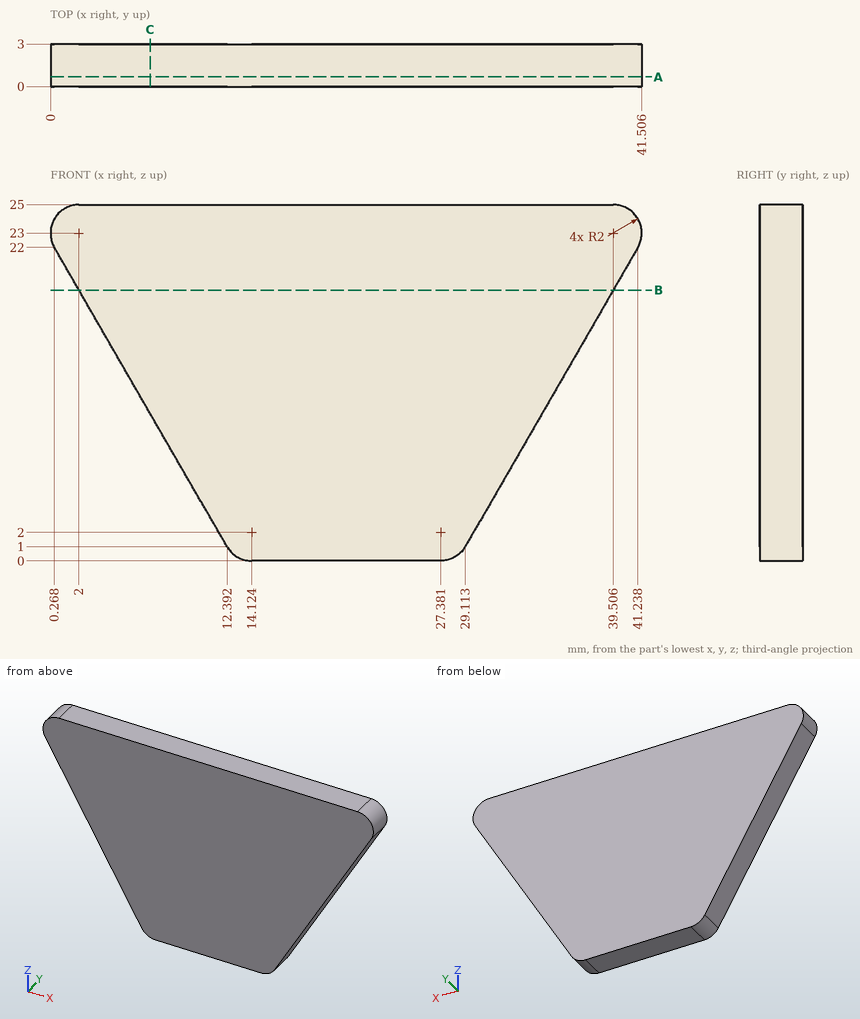
Design review of the part shown in the three views and the two pictorial views. Dimensions are in mm from the part's minimum x, y and z. Round coordinates to 2 decimals unless told otherwise and drop trailing zeros. Loops run counter-clockwise (first coordinate to the right, second up) from the corner with the lowest first, then second, coordinate; pieces in that order, holes last. Notation, with made-up numbers: (48.5, -2.75) - (105.5, -2.75) arc R16 ccw to (105.5, 5.25) - close; hole circle Ø9 at (22, -35). An arc over 180 degrees is marked (long way). Answer as CSV lines item,"result".
(1) Consider section B-B on z = 19. Give the boundary of the cut face in (x, y) (1 decimal).
Checked values:
outline,"(2, 0) - (39.5, 0) - (39.5, 3) - (2, 3) - close"
(2) Insertion check: P1, Ø1, axis at x = 29.5, y = 1.5, coming from the -Z side (1 decimal); P2, Ø3, axis at x = 17, z = 10.5, coming from the -Y side. Each pin has a flat end and moves straight along its axis. Give the tip position at first contact, or say it passes through.
Checked values:
P1,"stops at z = 0.8"
P2,"stops at y = 0"
(3) Wall thickness on line 1 (X direction, y = 2.6, z = 22); line 2 (Z direction, x = 31, y = 1.2) (1 decimal); line 3 (X direction, y = 1.15, z = 15.5) (1 decimal): over which ranges is each line inside the solid? List them lowest first.
Checked values:
line 1,"x = 0.27 to 41.24"
line 2,"z = 4.3 to 25"
line 3,"x = 4 to 37.5"
(4) Consider section A-A on y = 0.7. Give the boundary of the cut face in (x, z) (1 decimal), then the cut area to 3 significant figures.
Checked values:
outline,"(0.3, 22) - (12.4, 1) arc R2 ccw to (14.1, 0) - (27.4, 0) arc R2 ccw to (29.1, 1) - (41.2, 22) arc R2 ccw to (39.5, 25) - (2, 25) arc R2 ccw to start"
area,"744 mm2"
(5) Consider section C-C on x = 7. Give the boundary of the cut face in (y, z).
Checked values:
outline,"(0, 10.34) - (3, 10.34) - (3, 25) - (0, 25) - close"
